```python
from build123d import *

# Parameters (mm, degrees)
CROSSRECESS_DEPTH = 0.825
DRAFT9_ANGLE      = 30
FILLET5_R         = 0.3


with BuildPart() as part:
    # Sketch1 → Base (revolve)
    with BuildSketch(Plane.XY, mode=Mode.PRIVATE) as base_sk:
        Polygon((20, 1.5), (2.65, 1.5), (1.65, 1.5), (0.55, 2.6), (0, 2.6), (0, 0), (20, 0), align=None)
    revolve(base_sk.sketch.rotate(Axis((4.515812911, 0, 0), (-1, 0, 0)), 90), axis=Axis((4.515812911, 0, 0), (-1, 0, 0)))

    # Sketch6 → CrossRecess (cut)
    with BuildSketch(Plane(origin=(0, 0, 0), x_dir=(0, 0, -1), z_dir=(1, 0, 0))):
        Polygon((0.32, 0.32), (0.32, 1.6), (-0.32, 1.6), (-0.32, 0.32), (-1.6, 0.32), (-1.6, -0.32), (-0.32, -0.32), (-0.32, -1.6), (0.32, -1.6), (0.32, -0.32), (1.6, -0.32), (1.6, 0.32), align=None)
    extrude(amount=CROSSRECESS_DEPTH, mode=Mode.SUBTRACT)

    # Draft9
    draft9_faces = [part.faces().sort_by_distance(p)[0] for p in [
        (0.4125, 1.6, 0),
        (0.4125, 0, 1.6),
        (0.4125, -1.6, 0),
        (0.4125, 0, -1.6),
    ]]
    draft(draft9_faces, Plane(origin=(0, 2.6, 0), x_dir=(0, 0, -1), z_dir=(-1, 0, 0)), DRAFT9_ANGLE)

    # Fillet5
    fillet5_edges = [part.edges().sort_by_distance(p)[0] for p in [
        (0.4125, 0.32, 0.32),
        (0.4125, -0.32, 0.32),
        (0.4125, -0.32, -0.32),
        (0.4125, 0.32, -0.32),
    ]]
    fillet(fillet5_edges, radius=FILLET5_R)


solid = part.part
```
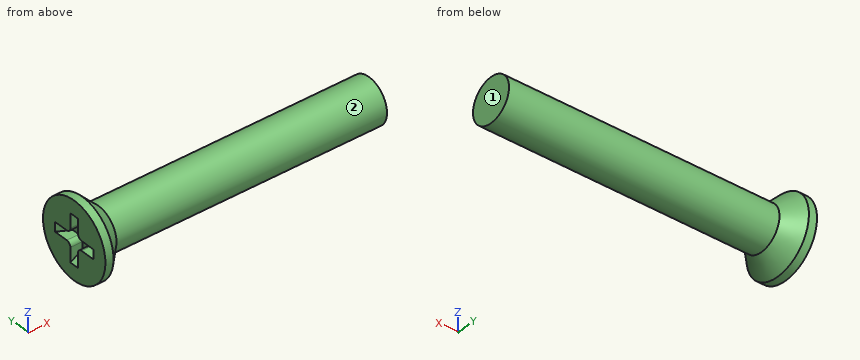
Verification items for the finished model (mm, model axes). Face numbers are marked on the shaded views. A direction names the side the tool comes from. Coordinates: 2 decimals unless noted, no trailing zeros. Write each loop counter-clockwise with the first axis right and the second up, starting at its lowest first coordinate (ties: lowest second). Pieces come first, ordered by that corner, then holes. Notation, with made-up numbers: (-3, 6) - (24, 6) arc R18 cw to (24, 14) - close; hole circle Ø7 at (86.5, 55). An arc over 180 degrees is marked (long way). One line per question, with ' | ' between items. Start each with the question number.
1. Access from +Z, -Z, +X, -X, +Y, -Y to the whole of each face (thin tool, end or side, straight path). Record for the marked faces 1 and 2.
2. Material ranges on line 1 along X through (y, z) = (0.2, -0.65) (3 decimals); line 2 along X through (y, z) = (-1.9, 0.75); line 3 along Y through (x, z) = (10, 1.35), recorded low to high.
3. Section check C-C (x = 6). Enter the section's corners in (y, z), plus the area to 3 significant figures.
4. Section check A-A (z = 0). Enter the section's corners in (x, y) (3 decimals).
5. Gauge pin test, flat ends, axial feed: P1, Ø0.7, axis at x = 0.5, z = 1.5, coming from the -Y side; P2, Ø3, axis at x = 14.5, y = -1, coming from the -Z side; P3, Ø0.7, axis at x = 0, z = -1, coming from the -Y side. Record the tip position at first contact, or that the pin passes through.
Computed values:
1) face 1: +Z, -Z, +X, +Y, -Y | face 2: +X
2) line 1: 0.825 to 20 | line 2: 0 to 1.11 | line 3: -0.65 to 0.65
3) outline: circle Ø3 at (0, 0) | area: 7.07 mm²
4) outline: (0, -2.6) - (0.55, -2.6) - (1.65, -1.5) - (20, -1.5) - (20, 1.5) - (1.65, 1.5) - (0.55, 2.6) - (0, 2.6) - (0, 1.6) - (0.825, 1.124) - (0.825, -1.124) - (0, -1.6) - close
5) P1: y = -2.33 | P2: z = -1.5 | P3: y = -2.52
